Autodesk Inventor part; units mm, degrees
ref_plane "YZ Plane" through (0, 0, 0) normal (1, 0, 0) x (0, 1, 0)
ref_plane "XZ Plane" through (0, 0, 0) normal (0, 1, 0) x (-1, 0, 0)
ref_plane "XY Plane" through (0, 0, 0) normal (0, 0, 1) x (1, 0, 0)
sketch "Sketch1" plane through (0, 0, 0) normal (0, 1, 0) x (-1, 0, 0)
  line L0 (0, 0) -> (65, 0)
  line L1 (65, 0) -> (65, -50)
  line L2 (65, -50) -> (0, -50)
  line L3 (0, -50) -> (0, 0)
  circle A0 centre (37.5, -25) radius 12.7
  dimension "d0" = 65
  dimension "d1" = 50
  dimension "d2" = 25.4
  dimension "d3" = 27.5
extrude "Extrusion1" add sketch "Sketch1" along normal blind 5.65
thread "Thread1"
sketch "Sketch2" plane through (0, 5.65, 0) normal (0, 1, 0) x (1, 0, 0)
  line L0 (-65, 0) -> (0, 0)
  line L1 (-65, 50) -> (-65, 0)
  line L2 (0, 0) -> (0, 50)
  line L3 (0, 50) -> (-65, 50)
  point P0 (-61.5, 3.5)
  point P1 (-3.5, 3.5)
  point P2 (-3.5, 46.5)
  point P3 (-61.5, 46.5)
  dimension "d15" = 3.5
  dimension "d16" = 3.5
  dimension "d17" = 3.5
  dimension "d18" = 3.5
  dimension "d19" = 3.5
  dimension "d20" = 3.5
  dimension "d21" = 3.5
  dimension "d22" = 3.5
hole "Hole1" at (-61.5, 5.65, -3.5) at (-3.5, 5.65, -3.5) at (-3.5, 5.65, -46.5) at (-61.5, 5.65, -46.5) direction (0, -1, 0) diameter 3.5 end through all
sketch "Sketch3" plane through (-65, 0, 0) normal (0, 0, 1) x (1, 0, 0)
  line L0 (14.8, 5.65) -> (40.2, 5.65)
  line L1 (27.5, 5.65) -> (27.5, 7.4)
  circle A0 centre (27.5, 7.4) radius 3.175
  circle A1 centre (27.5, 7.4) radius 6.35
  point P0 (65, 0)
  point P1 (21.3959, 5.65)
  point P2 (33.6041, 5.65)
  point P3 (30.1492, 5.65)
  point P4 (24.8508, 5.65)
  dimension "d23" = 1.75
  dimension "d24" = 6.35
  dimension "d25" = 12.7
extrude "Extrusion2" cut sketch "Sketch3" against normal blind 60 contours A0 L0 | L0 A0
extrude "Extrusion3" cut sketch "Sketch3" against normal blind 3.5 contours L0 A0 A1 picked at (22.7391, 5.1926)
sketch "Sketch4" plane through (0, 0, -50) normal (0, 0, -1) x (-1, 0, 0)
  arc A0 (34.8508, 5.65) -> (40.1492, 5.65) centre (37.5, 7.4) ccw
  circle A1 centre (37.5, 7.4) radius 6.35
  point P0 (0, 0)
  dimension "d30" = 12.7
extrude "Extrusion4" cut sketch "Sketch4" against normal blind 3.5
thread "Thread2"
equation "\"d30\" = d25"
properties part number "CuvetteHolderFace" material "Aluminum 6061"
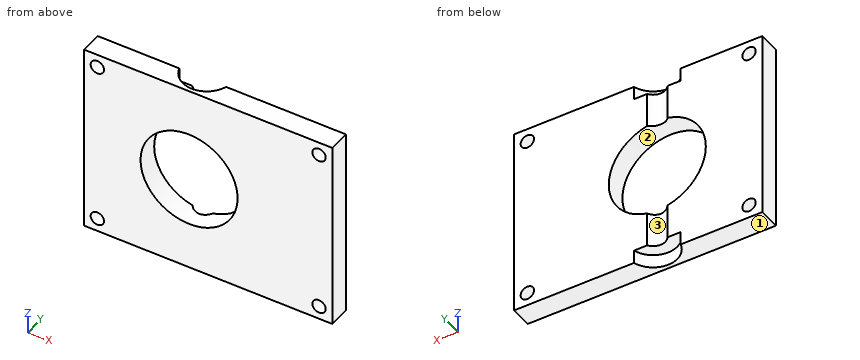
CAD build for the part. Positions are in the model's coordinates, mm. Face numbers are marked on the shaded views. Give positions to 0.01 mm unless a question says otherwise; leave off trailing zeros. Order: outer loops, then holes, each group sorted by start corner. A loop starts at its lowest first (then second) coordinate and runs counter-clockwise, first axis right, second up. Notation, with made-up numbers: (52, 21) -> (58, 21) arc R26 cw to (58, 49) -> close; hole circle Ø3 at (68, 45). An arc over 180 degrees is marked (long way). Return JSON: item names as keys, results as strings.
Q1. Saw through at C-C (x = -61.5). Write the cut outline in (y, z).
Working result:
{"outline": "(0, -50) -> (5.65, -50) -> (5.65, -48.25) -> (0, -48.25) -> close; (0, -44.75) -> (5.65, -44.75) -> (5.65, -5.25) -> (0, -5.25) -> close; (0, -1.75) -> (5.65, -1.75) -> (5.65, 0) -> (0, 0) -> close"}
Q2. Saw through at A-A (x = -37.5). Write the cut outline in (y, z) (3 decimals), then the cut area to 3 significant figures.
Working result:
{"outline": "(0, -50) -> (1.05, -50) -> (1.05, -46.5) -> (4.225, -46.5) -> (4.225, -37.7) -> (0, -37.7) -> close; (0, -12.3) -> (4.225, -12.3) -> (4.225, -3.5) -> (1.05, -3.5) -> (1.05, 0) -> (0, 0) -> close", "area": "81.7 mm²"}
Q3. Saw through at B-B (z = -25). Write the cut outline in (x, y).
Working result:
{"outline": "(-65, 0) -> (-50.2, 0) -> (-50.2, 5.65) -> (-65, 5.65) -> close; (-24.8, 0) -> (0, 0) -> (0, 5.65) -> (-24.8, 5.65) -> close"}
Q4. Saw through at D-D (y = 3.05). Write the cut outline in (x, z).
Working result:
{"outline": "(-65, -50) -> (-42.13, -50) -> (-42.13, -46.5) -> (-32.87, -46.5) -> (-32.87, -50) -> (0, -50) -> (0, 0) -> (-32.87, 0) -> (-32.87, -3.5) -> (-42.13, -3.5) -> (-42.13, 0) -> (-65, 0) -> close; hole circle Ø3.5 at (-61.5, -46.5); hole circle Ø3.5 at (-61.5, -3.5); hole circle Ø25.4 at (-37.5, -25); hole circle Ø3.5 at (-3.5, -46.5); hole circle Ø3.5 at (-3.5, -3.5)"}
Q5. Flat gauge pins, fed straight in: pin 1 (2 mm diameter, centred on x = -3.5, z = -3.5, fed in from -Y); pin 2 (1.5 mm diameter, centred on x = -37, y = 4, fed in from +Z); pin 3 (4.5 mm diameter, centred on x = -3.5, z = -46.5, fed in from -Y). Where does each tip first touch, or does it go through?
Working result:
{"pin 1": "through", "pin 2": "z = -3.5", "pin 3": "y = 0"}
Q6. Drill centre lines: line 1 (Z direction, x = -61.5, y = 1.9); line 2 (X direction, y = 1.85, z = -25.5); line 3 (X direction, y = 3.4, z = -30.5). Where is each one in solid material? Low to high.
Working result:
{"line 1": "-50 to -48.25, -44.75 to -5.25, -1.75 to 0", "line 2": "-65 to -50.19, -24.81 to 0", "line 3": "-65 to -48.95, -26.05 to 0"}
Q7. Mould opens along Z. For the marked faces 1, 2 and 3 say: pulls with the +Z half, pulls with the -Z half, needs draft (parallel to the pull), parting line crosses it, or undercut.
Working result:
{"face 1": "pulls with the -Z half", "face 2": "undercut", "face 3": "needs draft"}
